Check sheet for the modelled part. Datum: model origin and axes. Units: mm. Round coordinates to 2 decimals unless told otherwise and drop trailing zeros. Order: outer loops, then holes, each group sorted by start corner. A loop starts at its lowest first (then second) coordinate and runs counter-clockwise, first axis right, second up.
(1) Sectioned sample at D-D, the plane x = -6.35. Enter the section's corners in (y, z) (3 decimals).
(2) Sectioned sample at A-A, the plane x = 50.8. Enter the section's corners in (y, z) (3 decimals).
(3) Sectioned sample at B-B, the plane y = -565.15. Enter the section's corners in (x, z) (3 decimals), and give its area (3 significant figures).
(4) Mould release check, pull along Y, two halves, no side actions. Record for faces 1 (the cylindrical face through (6.95, -544.21, 1.57)), 2 (the flat face through (26, -584.2, 2)), 3 (the flat face through (17, -544, 3.175)): released by +Y, released by -Y, zero draft, split by the parting line, or undercut.
(5) Sectioned sample at C-C, the plane z = 1.55. Count the separate pieces of the cut face and the enclosed holes in it, and give its area (3 significant figures).
(6) Thickness scan on probe 1 along X at (y, z) = (-571.5, 1.65); probe 2 along X at (y, z) = (-577.85, 2.55); probe 3 along X at (y, z) = (-546.1, 1.05). Record the ranges inside material, lowest first.
```python
from build123d import *

# Parameters (mm, degrees)
BOSS_EXTRUDE1_DEPTH              = 3.175
F_97_0_0059_DIAMETER_HOLE1_D     = 3.96875
F_97_0_0059_DIAMETER_HOLE1_DEPTH = 6.349
F_97_0_0059_DIAMETER_HOLE1_TIP   = 1.192332791


with BuildPart() as part:
    # Sketch1 (on Front Plane) → Boss-Extrude1 (new body)
    with BuildSketch(Plane.XY):
        Polygon((-12.7, -584.2), (-12.7, -482.6), (12.7, -482.6), (63.5, -558.8), (63.5, -584.2), align=None)
    extrude(amount=BOSS_EXTRUDE1_DEPTH)

    # #97 (0.0059) Diameter Hole1
    with Locations(Plane(origin=(-12.7, -584.2, 3.175), x_dir=(0, -1, 0), z_dir=(0, 0, 1))):
        with Locations((-88.9, 6.35), (-88.9, 19.05), (-76.2, 12.7), (-63.5, 6.35), (-63.5, 19.05), (-50.8, 12.7), (-38.1, 6.35), (-38.1, 19.05), (-6.35, 12.7), (-19.05, 12.7), (-12.7, 25.4), (-19.05, 38.1), (-6.35, 38.1), (-12.7, 50.8), (-19.05, 63.5), (-6.35, 63.5)):
            Hole(F_97_0_0059_DIAMETER_HOLE1_D / 2, depth=F_97_0_0059_DIAMETER_HOLE1_DEPTH)
            with Locations((0, 0, -(F_97_0_0059_DIAMETER_HOLE1_DEPTH + F_97_0_0059_DIAMETER_HOLE1_TIP / 2))):  # 118° drill point
                Cone(0, F_97_0_0059_DIAMETER_HOLE1_D / 2, F_97_0_0059_DIAMETER_HOLE1_TIP, mode=Mode.SUBTRACT)


solid = part.part
```
Derived:
1. outline: (-584.2, 0) - (-548.084, 0) - (-548.084, 3.175) - (-584.2, 3.175) - close; (-544.116, 0) - (-522.684, 0) - (-522.684, 3.175) - (-544.116, 3.175) - close; (-518.716, 0) - (-497.284, 0) - (-497.284, 3.175) - (-518.716, 3.175) - close; (-493.316, 0) - (-482.6, 0) - (-482.6, 3.175) - (-493.316, 3.175) - close
2. outline: (-584.2, 0) - (-579.834, 0) - (-579.834, 3.175) - (-584.2, 3.175) - close; (-575.866, 0) - (-567.134, 0) - (-567.134, 3.175) - (-575.866, 3.175) - close; (-563.166, 0) - (-539.75, 0) - (-539.75, 3.175) - (-563.166, 3.175) - close
3. outline: (-12.7, 0) - (-1.984, 0) - (-1.984, 3.175) - (-12.7, 3.175) - close; (1.984, 0) - (23.416, 0) - (23.416, 3.175) - (1.984, 3.175) - close; (27.384, 0) - (48.816, 0) - (48.816, 3.175) - (27.384, 3.175) - close; (52.784, 0) - (63.5, 0) - (63.5, 3.175) - (52.784, 3.175) - close
3. area: 204 mm2
4. face 1: undercut
4. face 2: released by -Y
4. face 3: zero draft
5. separate pieces: 1
5. enclosed holes: 16
5. area: 5,610 mm2
6. probe 1: x = -12.7 to 10.72, 14.68 to 36.12, 40.08 to 63.5
6. probe 2: x = -12.7 to -1.98, 1.98 to 23.42, 27.38 to 48.82, 52.78 to 63.5
6. probe 3: x = -12.7 to -8.33, -4.37 to 4.37, 8.33 to 55.03
